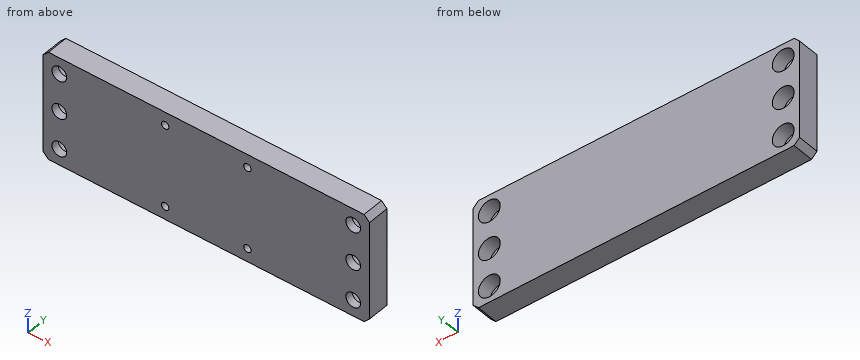
from build123d import *

# Parameters (mm, degrees)
SKETCH1_W                                            = 300
SKETCH1_H                                            = 100
BOSS_EXTRUDE1_DEPTH                                  = 20
CBORE_FOR_M12_HEXAGON_SOCKET_HEAD_CAP_SC_D           = 13.5
CBORE_FOR_M12_HEXAGON_SOCKET_HEAD_CAP_SC_CBORE_D     = 20
CBORE_FOR_M12_HEXAGON_SOCKET_HEAD_CAP_SC_CBORE_DEPTH = 13
CHAMFER1_SIZE                                        = 5
M8_TAPPED_HOLE1_D                                    = 6.8
M8_TAPPED_HOLE1_DEPTH                                = 15
M8_TAPPED_HOLE1_TIP                                  = 2.042926105


with BuildPart() as part:
    # Sketch1 → Boss-Extrude1 (new body)
    with BuildSketch(Plane(origin=(0, 0, 0), x_dir=(1, 0, 0), z_dir=(0, 1, 0))):
        Rectangle(SKETCH1_W, SKETCH1_H)
    extrude(amount=BOSS_EXTRUDE1_DEPTH)

    # CBORE for M12 Hexagon socket head cap screws1 (through all)
    with Locations(Plane(origin=(0, 20, 0), x_dir=(1, 0, 0), z_dir=(0, 1, 0))):
        with Locations((-135, 35), (-135, -35), (-135, 0), (135, 0), (135, -35), (135, 35)):
            CounterBoreHole(CBORE_FOR_M12_HEXAGON_SOCKET_HEAD_CAP_SC_D / 2, CBORE_FOR_M12_HEXAGON_SOCKET_HEAD_CAP_SC_CBORE_D / 2, CBORE_FOR_M12_HEXAGON_SOCKET_HEAD_CAP_SC_CBORE_DEPTH)

    # Chamfer1
    chamfer1_edges = [part.edges().sort_by_distance(p)[0] for p in [
        (-150, 10, -50),
        (150, 10, -50),
        (150, 10, 50),
        (-150, 10, 50),
    ]]
    chamfer(chamfer1_edges, length=CHAMFER1_SIZE)

    # M8 Tapped Hole1
    with Locations(Plane(origin=(0, 0, 0), x_dir=(-1, 0, 0), z_dir=(0, -1, 0))):
        with Locations((-37.8, 37.8), (37.8, 37.8), (37.8, -37.8), (-37.8, -37.8)):
            Hole(M8_TAPPED_HOLE1_D / 2, depth=M8_TAPPED_HOLE1_DEPTH)
            with Locations((0, 0, -(M8_TAPPED_HOLE1_DEPTH + M8_TAPPED_HOLE1_TIP / 2))):  # 118° drill point
                Cone(0, M8_TAPPED_HOLE1_D / 2, M8_TAPPED_HOLE1_TIP, mode=Mode.SUBTRACT)


solid = part.part
Geometry check sheet. Reference: the model listing, model coordinates, mm. Give positions to 0.01 mm unless a question says otherwise; leave off trailing zeros. Write each loop counter-clockwise with the first axis right and the second up, starting at its lowest first coordinate (ties: lowest second). Pieces come first, ordered by that corner, then holes. Notation, with made-up numbers: M 88,3.5 L 98,3.5 A21 cw 98,18.5 Z; hole C 85,77.5 d7. An arc over 180 degrees is marked long. Answer as CSV lines item,"result". Start each with the question number.
Q1. Material ranges on L1, parallel to Z at x = 37.8, y = 9.5; L2, parallel to Z at x = -135, y = 5; L3, parallel to Z at x = 135, y = 13.25, recorded low to high.
Q2. Go/stop test with flat-tipped pins: pin 1 (12 mm diameter, centred on x = -135, z = 35, fed in from -Y); pin 2 (16 mm diameter, centred on x = -135, z = 35, fed in from +Y); pin 3 (6 mm diameter, centred on x = 37.8, z = 37.8, fed in from -Y). Record where each tip stops, or that it passes through.
Q3. Section check A-A, the plane z = 3. Record the cut outline in (x, y), then the cut area to 3 significant figures.
Geometry says:
1,L1,"-50 to -41.2, -34.4 to 34.4, 41.2 to 50"
1,L2,"-50 to -41.75, -28.25 to -6.75, 6.75 to 28.25, 41.75 to 50"
1,L3,"-50 to -45, -25 to -10, 10 to 25, 45 to 50"
2,pin 1,"through"
2,pin 2,"y = 7"
2,pin 3,"y = 15.24"
3,outline,"M -150,0 L -141.05,0 L -141.05,7 L -144.54,7 L -144.54,20 L -150,20 Z; M -128.95,0 L 128.95,0 L 128.95,7 L 125.46,7 L 125.46,20 L -125.46,20 L -125.46,7 L -128.95,7 Z; M 141.05,0 L 150,0 L 150,20 L 144.54,20 L 144.54,7 L 141.05,7 Z"
3,area,"5,330 mm^2"
